from build123d import *

# Parameters (mm, degrees)
SKETCH1_R           = 2.38125
BOSS_EXTRUDE1_DEPTH = 3.175


with BuildPart() as part:
    # Sketch1 → Boss-Extrude1 (new body)
    with BuildSketch(Plane(origin=(0, 0, 0), x_dir=(1, 0, 0), z_dir=(0, 1, 0))):
        Polygon((0, 67.31), (0, 0), (25.4, 0), (25.4, 45.757385309), (49.492614691, 69.85), (95.25, 69.85), (95.25, 95.25), (33.02, 95.25), (33.02, 74.93), (25.4, 67.31), align=None)
        with Locations((12.7, 19.05)):
            Circle(SKETCH1_R, mode=Mode.SUBTRACT)
        with Locations((12.7, 31.75)):
            Circle(SKETCH1_R, mode=Mode.SUBTRACT)
        with Locations((12.7, 44.45)):
            Circle(SKETCH1_R, mode=Mode.SUBTRACT)
        with Locations((12.7, 57.15)):
            Circle(SKETCH1_R, mode=Mode.SUBTRACT)
        with Locations((38.1, 82.55)):
            Circle(SKETCH1_R, mode=Mode.SUBTRACT)
        with Locations((50.8, 82.55)):
            Circle(SKETCH1_R, mode=Mode.SUBTRACT)
        with Locations((63.5, 82.55)):
            Circle(SKETCH1_R, mode=Mode.SUBTRACT)
        with Locations((76.2, 82.55)):
            Circle(SKETCH1_R, mode=Mode.SUBTRACT)
        with Locations((88.9, 82.55)):
            Circle(SKETCH1_R, mode=Mode.SUBTRACT)
        with Locations((12.7, 6.35)):
            Circle(SKETCH1_R, mode=Mode.SUBTRACT)
    extrude(amount=BOSS_EXTRUDE1_DEPTH)


solid = part.part
Check sheet for the modelled part. Datum: model origin and axes. Units: mm. A direction names the side the tool comes from. Round coordinates to 2 decimals unless told otherwise and drop trailing zeros. Order: outer loops, then holes, each group sorted by start corner. A loop starts at its lowest first (then second) coordinate and runs counter-clockwise, first axis right, second up.
(1) Cross-section at B-B, the plane z = -6.35. Enter the section's corners in (x, y) (3 decimals).
(2) Go/stop test with a flat-tipped pin: P1, Ø1, axis at y = 1.5, z = -81.5, coming from the -X side. Record where the tip stops, or that it passes through.
(3) Access from +Z, -Z, +X, -X, +Y, -Y to the whole of each face (thin tool, end or side, straight path). Record for faces 1 (the cylindrical face through (62.984, 1.565, -80.225)), 2 (the flat face through (13, 2, -67.31)), 3 (the flat face through (72, 2, -69.85)).
(4) Draft check along Z on faces 4 (the flat face through (25.4, 2, -23)), 5 (the cylindrical face through (74.31, 1.57, -81.1)), 6 (the flat face through (29.26, 1.57, -71.17)). Enter one of: pulls with the +Z half, pulls with the -Z half, needs draft (parallel to the pull), parting line crosses it, or undercut.
(5) Cross-section at C-C, the plane y = 1.6. State how many separate pieces and enclosed holes the cut face has, and give its area (3 significant figures).
(6) Cross-section at D-D, the plane z = -77. Enter the section's corners in (x, y) (3 decimals).
(7) Scan lines: probe 1 along X at (y, z) = (1.2, -82.55); probe 2 along Z at (x, y) = (50.8, 2.3); probe 3 along X at (y, z) = (1.85, -44.5). Record each from-to range of solid material in increasing order.
(8) Cross-section at A-A, the plane x = 88.9. Enter the section's corners in (y, z) (3 decimals).
Check sheet entries:
1. outline: (0, 0) - (10.319, 0) - (10.319, 3.175) - (0, 3.175) - close; (15.081, 0) - (25.4, 0) - (25.4, 3.175) - (15.081, 3.175) - close
2. P1: stops at x = 33.02
3. face 1: +Y, -Y
3. face 2: -Z, -X, +Y, -Y
3. face 3: +Z, +X, +Y, -Y
4. face 4: needs draft
4. face 5: undercut
4. face 6: pulls with the -Z half
5. separate pieces: 1
5. enclosed holes: 10
5. area: 3,410 mm2
6. outline: (33.02, 0) - (95.25, 0) - (95.25, 3.175) - (33.02, 3.175) - close
7. probe 1: x = 33.02 to 35.72, 40.48 to 48.42, 53.18 to 61.12, 65.88 to 73.82, 78.58 to 86.52, 91.28 to 95.25
7. probe 2: z = -95.25 to -84.93, -80.17 to -69.85
7. probe 3: x = 0 to 10.32, 15.08 to 25.4
8. outline: (0, -95.25) - (3.175, -95.25) - (3.175, -84.931) - (0, -84.931) - close; (0, -80.169) - (3.175, -80.169) - (3.175, -69.85) - (0, -69.85) - close
